The listing builds one solid part. Answer for the finished solid, in the listing's coordinates (mm). A direction names the side the tool comes from. Coordinates: 2 decimals unless noted, no trailing zeros. Write each loop counter-clockwise with the first axis right and the second up, starting at its lowest first coordinate (ties: lowest second). Pieces come first, ordered by that corner, then holes.
(1) The part is cut by section A-A on z = 3. Give the number of separate pieces and of enclosed holes in the cut face, plus the area to 3 significant figures.
(2) For a pull along Y with two mould halves and no side action, classify faces 1 (the flat face through (-10.85, -5.34, 3.94)), 2 (the flat face through (2, 0, 0)), 3 (the cylindrical face through (-2.994, -22.804, 3.944)) as +Y half, -Y half, draft (parallel to the pull), parting line (faces both ways), or undercut.
(3) The part is cut by section B-B on y = -15.5. Determine the outline of the cut face in (x, z) (3 decimals), plus the area to 3 significant figures.
(4) Straight lines are drawn through the part: line 1 (Y direction, x = -7.5, z = 6.25); line 2 (X direction, y = 9.5, z = 7.25); line 3 (Y direction, x = 9, z = 7.5). For each, find the intervals that lie inside material, in ascending order.
(5) Which of the six approach directions +Z, -Z, +X, -X, +Y, -Y give full straight-line access (tool end or side, diameter ignored) to faces 4 (the cylindrical face through (1.418, -0.49, 3.796)), 5 (the conical face through (-1.53, -0.54, 7.82))?
(6) The part is cut by section C-C on y = 0. Determine the outline of the cut face in (x, z).
(7) The part is cut by section D-D on x = 7.5. Determine the outline of the cut face in (y, z), plus the area to 3 significant figures.
(8) Given P1, Ø1.1, axis at x = 0, z = 3, coming from the -Y side; P2, Ø1.5, axis at y = -7.5, z = 2, coming from the -X side; P3, Ø1.5, axis at y = 8, z = 4.5, coming from the -X side; P4, Ø10, axis at x = 10.5, y = 10, coming from the -Z side, each flat-ended and moving along its own axis, determine where each tip first touches the part or whether it passes through.
Autodesk Inventor part; units mm, degrees
ref_plane "YZ Plane" through (0, 0, 0) normal (1, 0, 0) x (0, 1, 0)
ref_plane "XZ Plane" through (0, 0, 0) normal (0, 1, 0) x (-1, 0, 0)
ref_plane "XY Plane" through (0, 0, 0) normal (0, 0, 1) x (1, 0, 0)
sketch "スケッチ1" plane through (0, 0, 0) normal (0, 0, 1) x (1, 0, 0)
  circle A0 centre (0, 0) radius 1.5
  circle A1 centre (0, 0) radius 3.1
  line L0 (-0.4, 0) -> (0.4, 0)
  line L1 (0.4, 0) -> (0.4, -3.1)
  line L2 (0.4, -3.1) -> (-0.4, -3.1)
  line L3 (-0.4, -3.1) -> (-0.4, 0)
  line L4 (-1.0712, 1.05) -> (1.0712, 1.05)
  circle A2 centre (0, 0) radius 23
  circle A3 centre (0, 0) radius 21.4
  line L5 (-1.4605, 1.0815) -> (-1.1105, 1.4385)
  line L6 (-1.1105, 1.4385) -> (0.175, 0.1785)
  line L7 (0.175, 0.1785) -> (-0.175, -0.1785)
  line L8 (-0.175, -0.1785) -> (-1.4605, 1.0815)
  line L9 (1.4605, 1.0815) -> (1.1105, 1.4385)
  line L10 (1.1105, 1.4385) -> (-0.175, 0.1785)
  line L11 (-0.175, 0.1785) -> (0.175, -0.1785)
  line L12 (0.175, -0.1785) -> (1.4605, 1.0815)
  line L13 (0, 0) -> (-1.0712, 1.05) construction
  line L14 (1.0712, 1.05) -> (0, 0) construction
  point P0 (0.4, -1.4457)
  point P1 (0.4, -3.0741)
  point P2 (-0.4, -3.0741)
  point P3 (-0.4, -1.4457)
  point P4 (-0.7141, 1.05)
  point P5 (0.7141, 1.05)
  point P6 (1.2312, 0.8568)
  point P7 (-1.2312, 0.8568)
  dimension "SHAFT_D" = 3
  dimension "SLIT" = 0.8
  dimension "HUB_THIN" = 1.6
  dimension "d3" = 1.05
  dimension "WHEEL_D" = 46
  dimension "d5" = 1.6
  dimension "d18" = 0.5
  dimension "d19" = 1.8
extrude "ハブ＆リム" add sketch "スケッチ1" along normal blind 8 contours A0 L12 L9 L10 L6 L5 L8 L3 A1 L1 | L10 L4 L6 A0 | A2
sketch "スケッチ2" plane through (0, 0, 0) normal (0, 0, 1) x (1, 0, 0)
  line L0 (-0.8, 2.6) -> (0.8, 2.6)
  line L1 (0.8, 2.6) -> (0.8, 21.4)
  line L2 (0.8, 21.4) -> (-0.8, 21.4)
  line L3 (-0.8, 21.4) -> (-0.8, 2.6)
  circle A0 centre (0, 0) radius 21.4
  point P0 (0, 21.4)
  dimension "d8" = 1.6
  dimension "d9" = 2.6
extrude "スポーク" add sketch "スケッチ2" along normal up to surface (8 mm away) contours L3 A0 L1 L0 | L3 L2 A0 | A0 L2 L1 picked at (0, 8.8667)
pattern_circular "円形状パターン1" count 3 over 360 about axis through (0, 0, -10) along (0, 0, 1) of "スポーク"
chamfer "面取り1" distance 0.3 angle 45 3 edges at (-1.4109, -0.5094, 8) (0, 1.05, 8) (1.4109, -0.5094, 8)
equation "\"d5\" = HUB_THIN"
properties part number "D-Shaft_Wheel2"
Model answer:
1. separate pieces: 1
1. enclosed holes: 3
1. area: 333 mm2
2. face 1: undercut
2. face 2: draft
2. face 3: parting line
3. outline: (-16.993, 0) - (-14.755, 0) - (-14.755, 8) - (-16.993, 8) - close; (14.755, 0) - (16.993, 0) - (16.993, 8) - (14.755, 8) - close
3. area: 35.8 mm2
4. line 1: y = -21.74 to -20.04, -5.25 to -3.41, 20.04 to 21.74
4. line 2: x = -20.95 to -19.18, -0.8 to 0.8, 19.18 to 20.95
4. line 3: y = -21.17 to -19.42, -6.12 to -4.27, 19.42 to 21.17
5. face 4: +Z, -Z
5. face 5: +Z
6. outline: (-23, 0) - (-21.4, 0) - (-21.4, 8) - (-23, 8) - close; (-3.1, 0) - (-1.5, 0) - (-1.5, 7.7) - (-1.8, 8) - (-3.1, 8) - close; (1.5, 0) - (3.1, 0) - (3.1, 8) - (1.8, 8) - (1.5, 7.7) - close; (21.4, 0) - (23, 0) - (23, 8) - (21.4, 8) - close
7. outline: (-21.74, 0) - (-20.04, 0) - (-20.04, 8) - (-21.74, 8) - close; (-5.25, 0) - (-3.41, 0) - (-3.41, 8) - (-5.25, 8) - close; (20.04, 0) - (21.74, 0) - (21.74, 8) - (20.04, 8) - close
7. area: 42.0 mm2
8. P1: stops at y = -23
8. P2: stops at x = -21.99
8. P3: stops at x = -21.83
8. P4: passes through
